Verification items for the finished model (mm, model axes). Round coordinates to 2 decimals unless told otherwise and drop trailing zeros. Write each loop counter-clockwise with the first axis right and the second up, starting at its lowest first coordinate (ties: lowest second). Pieces come first, ordered by that corner, then holes. Notation, with made-up numbers: M 80,43 L 107,43 A24 cw 107,81 Z; hole C 29,44.5 d8. An arc over 180 degrees is marked long. Write each question's results on one line, items separated by ' | '.
from build123d import *

# Parameters (mm, degrees)
F0_W     = 76.2
F0_H     = 244.288212
F0_R     = 19.053929
F1_DEPTH = 12.7


with BuildPart() as f1:
    # F0 (on Top) → F1 (new body)
    with BuildSketch(Plane.XY):
        with Locations((0.889241, -8.474177)):
            Rectangle(F0_W, F0_H)
        with Locations((0.889241, -8.474177)):
            Circle(F0_R, mode=Mode.SUBTRACT)
    extrude(amount=-F1_DEPTH)


solid = f1.part
1) Sectioned sample at B-B, the plane y = 5. Record the cut outline in (x, z), and give its area (3 significant figures).
Calculated:
outline: M -37.21,-12.7 L -12.58,-12.7 L -12.58,0 L -37.21,0 Z; M 14.36,-12.7 L 38.99,-12.7 L 38.99,0 L 14.36,0 Z | area: 626 mm²
2) Sectioned sample at C-C, the plane z = -8.5. Record the cut outline in (x, y).
Calculated:
outline: M -37.21,-130.62 L 38.99,-130.62 L 38.99,113.67 L -37.21,113.67 Z; hole C 0.89,-8.47 d38.11
3) Sectioned sample at A-A, the plane x = -3. Record the cut outline in (y, z).
Calculated:
outline: M -130.62,-12.7 L -27.13,-12.7 L -27.13,0 L -130.62,0 Z; M 10.18,-12.7 L 113.67,-12.7 L 113.67,0 L 10.18,0 Z
4) Depth check by flat-ended pin: P1, Ø6, axis at x = -23, y = -20, coming from the +Z side; P2, Ø23, axis at x = 0.89, y = -8.47, coming from the +Z side. Enter the tip coordinate at first touch or a pass-through.
Calculated:
P1: stops at z = 0 | P2: passes through
5) Draft check along Y on faces 1 (the cylindrical face through (11.133, 7.592, -6.261)), 2 (the flat face through (26, -7, 0)), 3 (the flat face through (0, 113.67, -6)). Enter one of: pulls with the +Y half, pulls with the -Y half, needs draft (parallel to the pull), parting line crosses it, or undercut.
Calculated:
face 1: undercut | face 2: needs draft | face 3: pulls with the +Y half
6) Material ranges on line 1 (Y direction, x = 0.5, z = -8.25); line 2 (Y direction, x = -4.5, z = -1); line 3 (X direction, y = -16, z = -2.75), recorded low to high. Write a range as [from, to].
Calculated:
line 1: y = [-130.62, -27.52], [10.58, 113.67] | line 2: y = [-130.62, -26.75], [9.8, 113.67] | line 3: x = [-37.21, -16.62], [18.39, 38.99]
